Verification items for this drawing (mm, ordinates from the low corner). Round coordinates to 2 decimals unless told otherwise and drop trailing zeros. Order: outer loops, then holes, each group sorted by start corner. A loop starts at its lowest first (then second) coordinate and runs counter-clockwise, first axis right, second up. Notation, with made-up numbers: (11, 38) -> (43, 38) arc R18 ccw to (43, 48) -> close; hole circle Ø9 at (78, 53.5). An arc over 180 degrees is marked (long way). Use a Markdown table: item, result. Add a question column.
Item 1: Sectioned sample at B-B, the plane z = 25.5. Record the cut outline in (x, y), and give its area (3 significant figures).
Item 2: Sectioned sample at A-A, the plane y = 50. Record the cut outline in (x, z), and give its area (3 significant figures).
Item 3: Mould release check, pull along Y, two halves, no side actions. Record for the marked faces 1, 2, 3 and 4: pulls with the +Y half, pulls with the -Y half, needs draft (parallel to the pull), parting line crosses it, or undercut.
Item 4: Material ranges on probe 1 along Y at (x, z) = (50, 30.5); probe 2 along Y at (x, z) = (50, 18.85); probe 3 along Z at (x, y) = (83, 81), recorded low to high. Write a range as [from, to].
Item 5: Gauge pin test, flat ends, axial feed: pin 1 Ø1.5 at (x, y) = (71, 51.5) entering from -Z; pin 2 Ø10 at (x, z) = (26, 13) entering from -Y; pin 3 Ø12 at (x, y) = (53, 53.5) entering from +Z; pin 4 Ø12 at (y, z) = (77.5, 18.5) entering from +X. Record the tip position at first contact, or that the pin passes through.
Item 6: Sectioned sample at C-C, the plane z = 13. Record the cut outline in (x, y).
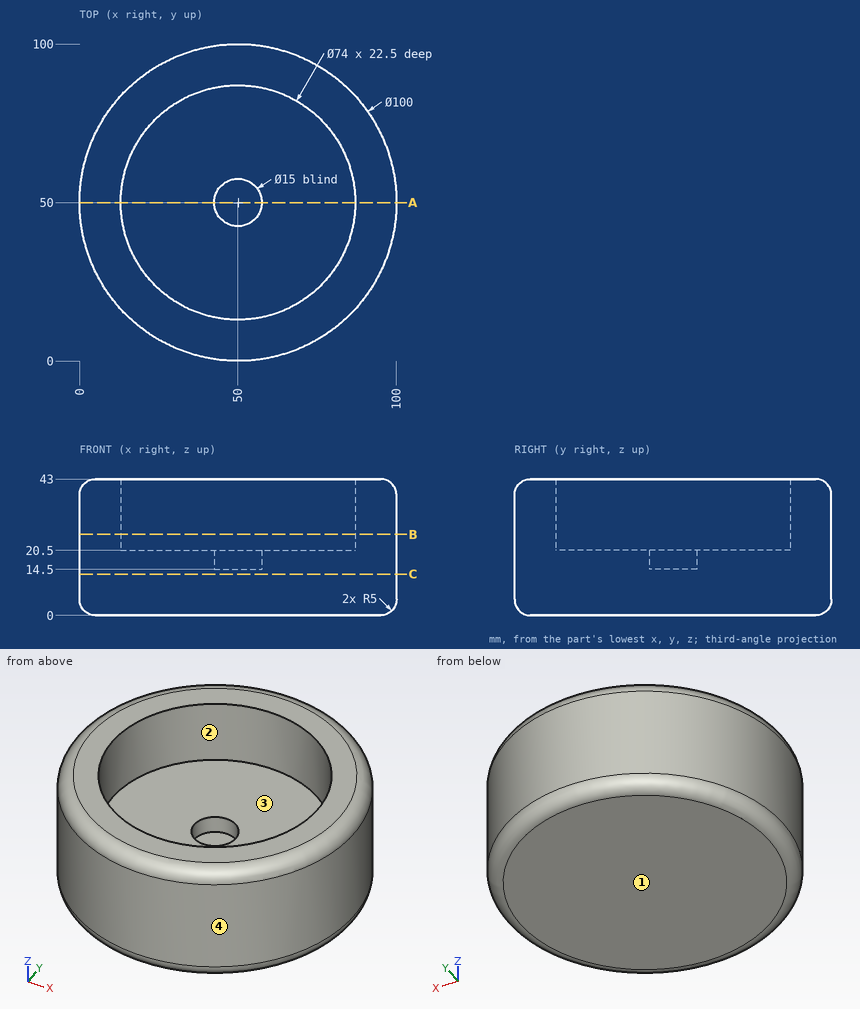
Found:
| question | item | result |
|---|---|---|
| 1 | outline | circle Ø100 at (50, 50); hole circle Ø74 at (50, 50) |
| 1 | area | 3,550 mm2 |
| 2 | outline | (0, 5) arc R5 ccw to (5, 0) -> (95, 0) arc R5 ccw to (100, 5) -> (100, 38) arc R5 ccw to (95, 43) -> (87, 43) -> (87, 20.5) -> (57.5, 20.5) -> (57.5, 14.5) -> (42.5, 14.5) -> (42.5, 20.5) -> (13, 20.5) -> (13, 43) -> (5, 43) arc R5 ccw to (0, 38) -> close |
| 2 | area | 2,520 mm2 |
| 3 | face 1 | needs draft |
| 3 | face 2 | undercut |
| 3 | face 3 | undercut |
| 3 | face 4 | parting line crosses it |
| 4 | probe 1 | y = [0, 13], [87, 100] |
| 4 | probe 2 | y = [0, 42.5], [57.5, 100] |
| 4 | probe 3 | z = [0.01, 42.99] |
| 5 | pin 1 | stops at z = 0 |
| 5 | pin 2 | stops at y = 3.75 |
| 5 | pin 3 | stops at z = 20.5 |
| 5 | pin 4 | stops at x = 95.14 |
| 6 | outline | circle Ø100 at (50, 50) |
